For this review, take the finished solid that the model builds, in its own axes (mm). A direction names the side the tool comes from. Coordinates: 2 decimals unless noted, no trailing zeros. Loops run counter-clockwise (first coordinate to the right, second up) from the corner with the lowest first, then second, coordinate; pieces in that order, holes last. Notation, with made-up numbers: (0.5, -36.5) - (41.5, -36.5) arc R24 cw to (41.5, -7.5) - close; hole circle Ø1 at (47, 9). An arc over 180 degrees is marked (long way). One line per item, written item: value. Start each with the question number.
1. The part is to be moulded in two halves that separate along Y. For faces 3 (the face through (18.6, 4.767, -3.9)), 4 (the face through (16.65, 1, -7)), 5 (the face through (17.917, 1.059, -12.914)), say which applies: released by +Y, released by -Y, zero draft, split by the parting line, or undercut.
2. For faces 1 (the face through (23.22, 0.67, 4.48)), 2 (the face through (22.7, 1.3, 3)), list the 3-axis set-ups (+Z, -Z, +X, -X, +Y, -Y) from which the entire face can be reached by the end or side of a thin tool; tool diameter is ignored.
3. Take a section at A-A, the plane x = 24.65. State the section outline as (y, z) points, and give its area (3 significant figures).
4. Take a section at B-B, the plane z = -4.5. State the section outline as (x, y) points, and give its area (3 significant figures).
5. Take a section at D-D, the plane x = 20.5. State the section outline as (y, z) points.
6. Take a section at C-C, the plane y = 0. State the section outline as (x, z) points, and give its area (3 significant figures).
7. To check wall thickness, follow line 1 (Z direction, x = 18.5, y = 2.5); line 2 (Y direction, x = 24.65, z = 4.8); line 3 (X direction, y = 0.5, z = 4.25). State the ranges of each line that lie inside material, in increasing order. Write a range as from..to.
8. Insertion check: pin 1 (3.5 mm diameter, centred on x = 24.65, y = 1.27, fed in from -Z). The pin has a flat end and moves straight along its axis. Give the tip position at first contact, or say it passes through.
```python
from build123d import *

# Parameters (mm, degrees)
SKETCH1_W           = 132
SKETCH1_H           = 160
BOSS_EXTRUDE1_DEPTH = 6
SKETCH3_W           = 32
SKETCH3_H           = 54
SKETCH3_W_2         = 26
SKETCH3_H_2         = 48
BOSS_EXTRUDE2_DEPTH = 17.5
SKETCH4_W           = 32
SKETCH4_H           = 54
BOSS_EXTRUDE3_DEPTH = 3
SKETCH5_W           = 25
SKETCH5_H           = 17
CUT_EXTRUDE1_DEPTH  = 3
SKETCH6_W           = 12
SKETCH6_H           = 54
BOSS_EXTRUDE4_DEPTH = 3
SKETCH7_R           = 1.6
CUT_EXTRUDE2_DEPTH  = 106.177231376
SKETCH8_W           = 3
SKETCH8_H           = 6.5
BOSS_EXTRUDE5_DEPTH = 20
SKETCH9_R           = 1.55
CUT_EXTRUDE3_DEPTH  = 6
SKETCH10_R          = 1.6
CUT_EXTRUDE4_DEPTH  = 108.043215572
SKETCH11_W          = 2.5
SKETCH11_H          = 7
BOSS_EXTRUDE6_DEPTH = 19.36
SKETCH12_R          = 1.6
CUT_EXTRUDE5_DEPTH  = 19.36
SKETCH13_W          = 3
SKETCH13_H          = 7
BOSS_EXTRUDE7_DEPTH = 15
SKETCH14_R          = 2
CUT_EXTRUDE6_DEPTH  = 15
CUT_EXTRUDE7_START  = -6
CUT_EXTRUDE7_DEPTH  = 6
SKETCH16_R          = 1.6
CUT_EXTRUDE8_DEPTH  = 15
SKETCH17_W          = 117.76
SKETCH17_H          = 77.767250212
CUT_EXTRUDE9_DEPTH  = 109
SKETCH18_R          = 1.55
CUT_EXTRUDE10_DEPTH = 109
SKETCH18_3_W        = 9
SKETCH18_3_H        = 7
CUT_EXTRUDE11_DEPTH = 3
SKETCH19_W          = 47.5
SKETCH19_H          = 6
CUT_EXTRUDE12_DEPTH = 80
SKETCH19_3_W        = 2.7
SKETCH19_3_H        = 6
CUT_EXTRUDE13_DEPTH = 80
SKETCH19_4_W        = 9
SKETCH19_4_H        = 3
CUT_EXTRUDE14_DEPTH = 80
SKETCH20_W          = 62.599740271
SKETCH20_H          = 63.599226712
CUT_EXTRUDE15_DEPTH = 80


# Read off the part's stored shape, not the designer's step: Cut-Extrude7
with BuildPart() as part:
    # Sketch1 → Boss-Extrude1 (new body)
    with BuildSketch(Plane.XY):
        Rectangle(SKETCH1_W, SKETCH1_H)
    extrude(amount=BOSS_EXTRUDE1_DEPTH)

    # Sketch3 → Boss-Extrude2 (add)
    with BuildSketch(Plane.XY.offset(6)):
        with Locations((0, -53)):
            Rectangle(SKETCH3_W, SKETCH3_H)
        with Locations((0, -53)):
            Rectangle(SKETCH3_W_2, SKETCH3_H_2, mode=Mode.SUBTRACT)
    extrude(amount=BOSS_EXTRUDE2_DEPTH)

    # Sketch4 → Boss-Extrude3 (add)
    with BuildSketch(Plane.XY.offset(23.5)):
        with Locations((0, -53)):
            Rectangle(SKETCH4_W, SKETCH4_H)
    extrude(amount=BOSS_EXTRUDE3_DEPTH)

    # Sketch5 → Cut-Extrude1 (cut)
    with BuildSketch(Plane.XZ.offset(80)):
        with Locations((0, 14.5)):
            Rectangle(SKETCH5_W, SKETCH5_H)
    extrude(amount=-CUT_EXTRUDE1_DEPTH, mode=Mode.SUBTRACT)

    # Sketch6 → Boss-Extrude4 (add)
    with BuildSketch(Plane.XY.offset(6)):
        with Locations((-22, -53)):
            Rectangle(SKETCH6_W, SKETCH6_H)
        with Locations((22, -53)):
            Rectangle(SKETCH6_W, SKETCH6_H)
    extrude(amount=BOSS_EXTRUDE4_DEPTH)

    # Sketch7 → Cut-Extrude2 (cut, through all)
    with BuildSketch(Plane.XY.offset(9)):
        with Locations((-22, -69)):
            Circle(SKETCH7_R)
        with Locations((-22, -33)):
            Circle(SKETCH7_R)
        with Locations(Location((22, -69, 0), (0, 0, 180))):
            Circle(SKETCH7_R)
        with Locations(Location((22, -33, 0), (0, 0, 180))):
            Circle(SKETCH7_R)
    extrude(amount=-CUT_EXTRUDE2_DEPTH, mode=Mode.SUBTRACT)

    # Sketch8 → Boss-Extrude5 (add)
    with BuildSketch(Plane.XY.offset(6)):
        with Locations((-54.38, -76.75)):
            Rectangle(SKETCH8_W, SKETCH8_H)
        with Locations((-54.38, -30.25)):
            Rectangle(SKETCH8_W, SKETCH8_H)
    boss_extrude5 = extrude(amount=BOSS_EXTRUDE5_DEPTH)

    # Sketch9 → Cut-Extrude3 (cut)
    with BuildSketch(Plane.ZY.offset(55.88)):
        with Locations((10.35, -76.75)):
            Circle(SKETCH9_R)
        with Locations((19.65, -76.75)):
            Circle(SKETCH9_R)
        with Locations((10.35, -30.25)):
            Circle(SKETCH9_R)
        with Locations((19.65, -30.25)):
            Circle(SKETCH9_R)
    cut_extrude3 = extrude(amount=-CUT_EXTRUDE3_DEPTH, mode=Mode.SUBTRACT)

    # Mirror1: Boss-Extrude5, Cut-Extrude3 across plane
    add(boss_extrude5.mirror(Plane(origin=(0, 0, 0), x_dir=(0, 0, 1), z_dir=(1, 0, 0))))
    add(cut_extrude3.mirror(Plane(origin=(0, 0, 0), x_dir=(0, 0, 1), z_dir=(1, 0, 0))), mode=Mode.SUBTRACT)

    # Sketch10 → Cut-Extrude4 (cut, through all)
    with BuildSketch(Plane(origin=(0, 0, 0), x_dir=(-1, 0, 0), z_dir=(0, 0, -1))):
        with Locations((-24.1, -75.572749788)):
            Circle(SKETCH10_R)
        with Locations((-21.15, -12.732749788)):
            Circle(SKETCH10_R)
        with Locations(Location((21.15, -12.732749788, 0), (0, 0, 180))):
            Circle(SKETCH10_R)
        with Locations((24.1, -75.572749788)):
            Circle(SKETCH10_R)
    extrude(amount=-CUT_EXTRUDE4_DEPTH, mode=Mode.SUBTRACT)

    # Sketch11 → Boss-Extrude6 (add)
    with BuildSketch(Plane(origin=(0, 0, 0), x_dir=(-1, 0, 0), z_dir=(0, 0, -1))):
        with Locations((-17.9, 1.267250212)):
            Rectangle(SKETCH11_W, SKETCH11_H)
        with Locations((-17.9, 50.267250212)):
            Rectangle(SKETCH11_W, SKETCH11_H)
    extrude(amount=BOSS_EXTRUDE6_DEPTH)

    # Sketch12 → Cut-Extrude5 (cut)
    with BuildSketch(Plane(origin=(19.15, 0, 0), x_dir=(0, 0, -1), z_dir=(1, 0, 0))):
        with Locations(Location((4.5, 50.267250212, 0), (0, 0, 90))):
            Circle(SKETCH12_R)
        with Locations(Location((14.5, 50.267250212, 0), (0, 0, 90))):
            Circle(SKETCH12_R)
        with Locations(Location((4.5, 1.267250212, 0), (0, 0, 90))):
            Circle(SKETCH12_R)
        with Locations(Location((14.5, 1.267250212, 0), (0, 0, 90))):
            Circle(SKETCH12_R)
    extrude(amount=-CUT_EXTRUDE5_DEPTH, mode=Mode.SUBTRACT)

    # Sketch13 → Boss-Extrude7 (add)
    with BuildSketch(Plane(origin=(0, 0, 0), x_dir=(-1, 0, 0), z_dir=(0, 0, -1))):
        with Locations((29.35, 35.967250212)):
            Rectangle(SKETCH13_W, SKETCH13_H)
    extrude(amount=BOSS_EXTRUDE7_DEPTH)

    # Sketch14 → Cut-Extrude6 (cut)
    with BuildSketch(Plane.ZY.offset(30.85)):
        with Locations((-9.9, 35.967250212)):
            Circle(SKETCH14_R)
    extrude(amount=-CUT_EXTRUDE6_DEPTH, mode=Mode.SUBTRACT)

    # Cut-Extrude7 outline → Cut-Extrude7 (cut)
    with BuildSketch(Plane(origin=(0, 0, 0), x_dir=(-1, 0, 0), z_dir=(0, 0, -1)).offset(CUT_EXTRUDE7_START)):
        Polygon((-30.85, 56.767250212), (30.85, 56.767250212), (30.85, -24), (58.88, -24), (58.88, -80), (66, -80), (66, 80), (-66, 80), (-66, -80), (-58.88, -80), (-58.88, -24), (-30.85, -24), align=None)
    extrude(amount=CUT_EXTRUDE7_DEPTH, mode=Mode.SUBTRACT)

    # Sketch16 → Cut-Extrude8 (cut)
    with BuildSketch(Plane(origin=(0, 0, 0), x_dir=(-1, 0, 0), z_dir=(0, 0, -1))):
        Circle(SKETCH16_R)
        with Locations((0, 52.767250212)):
            Circle(SKETCH16_R)
    extrude(amount=-CUT_EXTRUDE8_DEPTH, mode=Mode.SUBTRACT)

    # Sketch17 → Cut-Extrude9 (cut)
    with BuildSketch(Plane(origin=(0, 0, 0), x_dir=(-1, 0, 0), z_dir=(0, 0, -1))):
        with Locations((0, -41.116374894)):
            Rectangle(SKETCH17_W, SKETCH17_H)
    extrude(amount=-CUT_EXTRUDE9_DEPTH, mode=Mode.SUBTRACT)

    # Sketch18 → Cut-Extrude10 (cut)
    with BuildSketch(Plane(origin=(0, 0, 0), x_dir=(-1, 0, 0), z_dir=(0, 0, -1))):
        with Locations((-24.65, 1.267250212)):
            Circle(SKETCH18_R)
    extrude(amount=-CUT_EXTRUDE10_DEPTH, mode=Mode.SUBTRACT)

    # Sketch18<3> → Cut-Extrude11 (cut)
    with BuildSketch(Plane(origin=(0, 0, 0), x_dir=(-1, 0, 0), z_dir=(0, 0, -1))):
        with Locations((-23.65, 1.267250212)):
            Rectangle(SKETCH18_3_W, SKETCH18_3_H)
    extrude(amount=-CUT_EXTRUDE11_DEPTH, mode=Mode.SUBTRACT)

    # Sketch19 → Cut-Extrude12 (cut)
    with BuildSketch(Plane.XZ.offset(2.232749788)):
        with Locations((-7.1, 3)):
            Rectangle(SKETCH19_W, SKETCH19_H)
    extrude(amount=-CUT_EXTRUDE12_DEPTH, mode=Mode.SUBTRACT)


with BuildPart() as body_2:
    # of the pieces the cut leaves, the one that is kept (cut_extrude12_keep)
    add(part.part.solids().sort_by_distance((30.85, -2.232749788, 0))[0])

    # Sketch19<3> → Cut-Extrude13 (cut)
    with BuildSketch(Plane.XZ.offset(2.232749788)):
        with Locations((29.5, 3)):
            Rectangle(SKETCH19_3_W, SKETCH19_3_H)
    extrude(amount=-CUT_EXTRUDE13_DEPTH, mode=Mode.SUBTRACT)

    # Sketch19<4> → Cut-Extrude14 (cut)
    with BuildSketch(Plane.XZ.offset(2.232749788)):
        with Locations((23.65, 1.5)):
            Rectangle(SKETCH19_4_W, SKETCH19_4_H)
    extrude(amount=-CUT_EXTRUDE14_DEPTH, mode=Mode.SUBTRACT)

    # Sketch20 → Cut-Extrude15 (cut)
    with BuildSketch(Plane(origin=(0, 0, 0), x_dir=(-1, 0, 0), z_dir=(0, 0, -1))):
        with Locations((-47.949870136, 36.566863568)):
            Rectangle(SKETCH20_W, SKETCH20_H)
    extrude(amount=-CUT_EXTRUDE15_DEPTH, mode=Mode.SUBTRACT)


with BuildPart() as body_2_2:
    # of the pieces the cut leaves, the one that is kept (cut_extrude15_keep)
    add(body_2.part.solids().sort_by_distance((16.65, -2.232749788, -19.36))[0])


solid = body_2_2.part
```
Solutions:
1. face 3: released by +Y
1. face 4: zero draft
1. face 5: undercut
2. face 1: +Z, -Z
2. face 2: -Z, +X, +Y, -Y
3. outline: (-2.23, 3) - (-0.28, 3) - (-0.28, 6) - (-2.23, 6) - close; (2.82, 3) - (4.77, 3) - (4.77, 6) - (2.82, 6) - close
3. area: 11.7 mm2
4. outline: (16.65, -2.23) - (19.15, -2.23) - (19.15, -0.33) - (16.65, -0.33) - close; (16.65, 2.87) - (19.15, 2.87) - (19.15, 4.77) - (16.65, 4.77) - close
4. area: 9.50 mm2
5. outline: (-2.23, 3) - (4.77, 3) - (4.77, 6) - (-2.23, 6) - close
6. outline: (16.65, -19.36) - (19.15, -19.36) - (19.15, -15.48) - (16.65, -15.48) - close; (16.65, -13.52) - (19.15, -13.52) - (19.15, -5.48) - (16.65, -5.48) - close; (16.65, -3.52) - (19.15, -3.52) - (19.15, 3) - (23.76, 3) - (23.76, 6) - (16.65, 6) - close; (25.54, 3) - (28.15, 3) - (28.15, 6) - (25.54, 6) - close
6. area: 75.3 mm2
7. line 1: -19.36..-15.52, -13.48..-5.52, -3.48..6
7. line 2: -2.23..-0.28, 2.82..4.77
7. line 3: 16.65..23.3, 26..28.15
8. pin 1: z = 3
